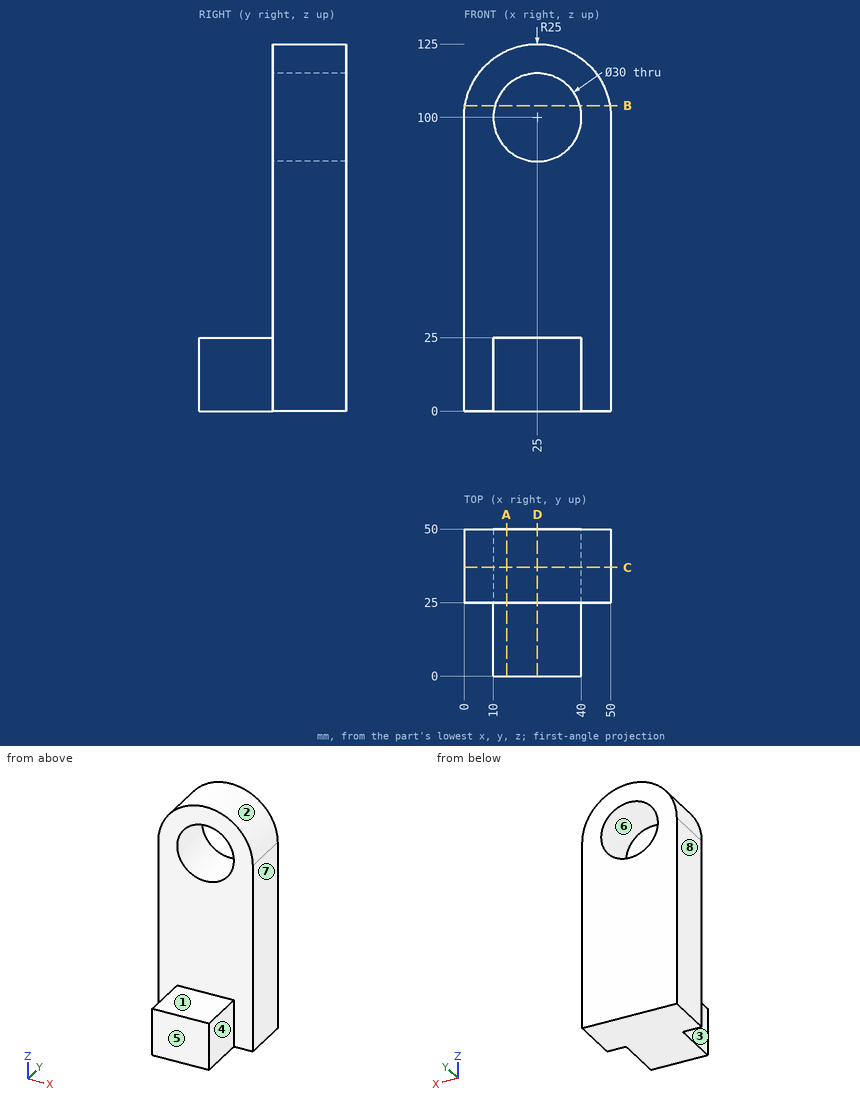
Can you work these out from the drawing? Everything is in mm from the part's minimum corner. A direction names the side the tool comes from. Give positions to 0.01 mm unless a question says otherwise; leave off trailing zeros. Loops run counter-clockwise (first coordinate to the right, second up) from the corner with the lowest first, then second, coordinate; pieces in that order, holes last. Notation, with made-up numbers: M 35.5,47 L 74.5,47 A33 ccw 74.5,78 Z; hole C 82,56.25 d2. An arc over 180 degrees is marked long. Use CSV: the item, a comma, the result in double quotes. Start each with the question number.
1. On a 3-axis mill with a long thin cutter (end or side, diameter ignored), from which of +Z, -Z, +X, -X, +Y, -Y can I reach the whole of each face in a straight line? I mean the marked faces 1, 2, 3 and 4. Say none if no direction works.
2. If we mould it in two halves opening along X, with no side actions, what happens to the marked faces 5, 6, 7 and 8? For each: released by +X, released by -X, zero draft, split by the parting line, or undercut.
3. If I drill on L1, parallel to Z at x = 25, y = 43.25; L2, parallel to Y at x = 16, z = 33.5; L3, parallel to X at y = 8, z = 8.5, over which ranges is the centre line in solid material (lowest first)?
4. Imagine slicing it at A-A, the plane x = 14.5. Write out the boundary of the cut face in (y, z), plus the area to 3 significant figures.
5. For P1, Ø10, axis at x = 6, y = 36.5, coming from the +Z side; P2, Ø12.5, axis at y = 8, z = 16, coming from the -X side; P3, Ø12.5, axis at y = 6.5, z = 18, coming from the +X side, each with a flat end and sliding along its axis, tell me the tip position at first contact or that it passes through.
6. Imagine slicing it at D-D, the plane x = 25. Write out the boundary of the cut face in (y, z).
7. Imagine slicing it at C-C, the plane y = 37. Write out the boundary of the cut face in (x, z).
8. Imagine slicing it at B-B, the plane z = 104. Write out the boundary of the cut face in (x, y).
Response values:
1,face 1,"+Z, +X, -X, -Y"
1,face 2,"+Z, +Y, -Y"
1,face 3,"+Z, -Z, -X, -Y"
1,face 4,"+Z, -Z, +X, -Y"
2,face 5,"zero draft"
2,face 6,"undercut"
2,face 7,"released by +X"
2,face 8,"released by -X"
3,L1,"0 to 85, 115 to 125"
3,L2,"25 to 50"
3,L3,"10 to 40"
4,outline,"M 0,0 L 50,0 L 50,89.29 L 25,89.29 L 25,25 L 0,25 Z; M 25,110.71 L 50,110.71 L 50,122.69 L 25,122.69 Z"
4,area,"3,160 mm^2"
5,P1,"z = 120.71"
5,P2,"x = 10"
5,P3,"x = 40"
6,outline,"M 0,0 L 50,0 L 50,85 L 25,85 L 25,25 L 0,25 Z; M 25,115 L 50,115 L 50,125 L 25,125 Z"
7,outline,"M 0,0 L 50,0 L 50,100 A25 ccw 0,100 Z; hole C 25,100 d30"
8,outline,"M 0.32,25 L 10.54,25 L 10.54,50 L 0.32,50 Z; M 39.46,25 L 49.68,25 L 49.68,50 L 39.46,50 Z"
